The listing builds one solid part. Answer for the finished solid, in the listing's coordinates (mm). A direction names the side the tool comes from. Coordinates: 2 decimals unless noted, no trailing zeros. Loops run counter-clockwise (first coordinate to the right, second up) from the corner with the lowest first, then second, coordinate; pieces in that order, holes last. Notation, with made-up numbers: (-38.5, 1.25) -> (-29.5, 1.25) arc R21 cw to (-29.5, 13.25) -> close; hole circle Ø10 at (67, 5). An arc over 180 degrees is marked (long way). Answer in a Markdown table with one row per item.
```python
from build123d import *

# Parameters (mm, degrees)
PAD016_DEPTH         = 27.5
POCKET034_DEPTH      = 185.6284208373
SKETCH105_W          = 70
SKETCH105_H          = 70
POCKET036_DEPTH      = 2.501
SKETCH114_W          = 70
SKETCH114_H          = 16
POCKET051_DEPTH      = 30.601
POCKET051_DEPTH_BACK = 30.601
PAD020_DEPTH         = 5
SKETCH134_R          = 2.3
SKETCH135_R          = 4
POCKET052_DEPTH      = 9
POCKET053_DEPTH      = 0.001
POCKET053_DEPTH_BACK = 22.501
SKETCH138_R          = 6.5
POCKET054_DEPTH      = 12.8357525158
POCKET056_DEPTH      = 2.5010001


with BuildPart() as part:
    # Sketch096 → Pad016 (new body)
    with BuildSketch(Plane.XY.offset(2.5)):
        with BuildLine():
            Line((-22.6, 30.6), (22.6, 30.6))
            ThreePointArc((30.6, 22.6), (28.2568542495, 28.2568542495), (22.6, 30.6))
            Line((30.6, 22.6), (30.6, -22.6))
            ThreePointArc((22.6, -30.6), (28.2568542495, -28.2568542495), (30.6, -22.6))
            Line((22.6, -30.6), (-22.6, -30.6))
            ThreePointArc((-30.6, -22.6), (-28.2568542495, -28.2568542495), (-22.6, -30.6))
            Line((-30.6, -22.6), (-30.6, 22.6))
            ThreePointArc((-22.6, 30.6), (-28.2568542495, 28.2568542495), (-30.6, 22.6))
        make_face()
    extrude(amount=-PAD016_DEPTH)

    # Sketch103 → Pocket034 (cut, through all)
    with BuildSketch(Plane.XY.offset(-1.5)):
        with BuildLine():
            Line((14.1, 7.65), (20.4, 7.65))
            ThreePointArc((21.9, 6.15), (21.4606601718, 7.2106601718), (20.4, 7.65))
            Line((21.9, 6.15), (21.9, -6.15))
            ThreePointArc((20.4, -7.65), (21.4606601718, -7.2106601718), (21.9, -6.15))
            Line((20.4, -7.65), (14.1, -7.65))
            ThreePointArc((12.6, -6.15), (13.0393398282, -7.2106601718), (14.1, -7.65))
            Line((12.6, -6.15), (12.6, 6.15))
            ThreePointArc((14.1, 7.65), (13.0393398282, 7.2106601718), (12.6, 6.15))
        make_face()
    pocket034 = extrude(amount=POCKET034_DEPTH, mode=Mode.SUBTRACT)

    # Mirrored008: Pocket034 across YZ
    add(pocket034.mirror(Plane.YZ), mode=Mode.SUBTRACT)

    # Sketch105 → Pocket036 (cut, through all)
    with BuildSketch(Plane.XY):
        Rectangle(SKETCH105_W, SKETCH105_H)
        with BuildLine():
            Line((-22.8, 25.9), (22.8, 25.9))
            ThreePointArc((26.3, 22.4), (25.2748737342, 24.8748737342), (22.8, 25.9))
            Line((26.3, 22.4), (26.3, -22.4))
            ThreePointArc((22.8, -25.9), (25.2748737342, -24.8748737342), (26.3, -22.4))
            Line((22.8, -25.9), (-22.8, -25.9))
            ThreePointArc((-26.3, -22.4), (-25.2748737342, -24.8748737342), (-22.8, -25.9))
            Line((-26.3, -22.4), (-26.3, 22.4))
            ThreePointArc((-22.8, 25.9), (-25.2748737342, 24.8748737342), (-26.3, 22.4))
        make_face(mode=Mode.SUBTRACT)
    extrude(amount=POCKET036_DEPTH, mode=Mode.SUBTRACT)

    # Sketch107 → Groove012 (revolve, cut)
    with BuildSketch(Plane.XZ):
        Polygon((19, -1.5), (21.8, -1.5), (21.2, -3.1484864517), (21.2, -13.5), (19, -13.5), align=None)
    groove012 = revolve(axis=Axis((19, 0, -1.5), (0, 0, 1)), mode=Mode.SUBTRACT)

    # Mirrored009: Groove012 across YZ
    add(groove012.mirror(Plane.YZ), mode=Mode.SUBTRACT)

    # Sketch114 → Pocket051 (cut, two sides)
    with BuildSketch(Plane.XZ) as pocket051_sk:
        with Locations((0, -18)):
            Rectangle(SKETCH114_W, SKETCH114_H)
    extrude(amount=-POCKET051_DEPTH, mode=Mode.SUBTRACT)
    extrude(pocket051_sk.sketch, amount=POCKET051_DEPTH_BACK, mode=Mode.SUBTRACT)

    # AdditivePipe004: sweep along a path in Sketch130
    with BuildLine(Plane.XY) as additivepipe004_path:
        Line((27, 16), (27, -5))
        ThreePointArc((27, -5), (25.1488749734, -9.9623583103), (20.5, -12.5))
        ThreePointArc((20.5, -12.5), (15.8511250266, -15.0376416897), (14, -20))
        Line((14, -20), (14, -30.6))
    # Sketch131 → AdditivePipe004 (sweep)
    with BuildSketch(Plane.XZ):
        with BuildLine():
            ThreePointArc((29.037037037, -18.5506966813), (27, -17.5), (24.962962963, -18.5506966813))
            ThreePointArc((24.6, -18.4347524158), (24.7391419381, -18.6252682846), (24.962962963, -18.5506966813))
            Line((24.6, -10), (24.6, -18.4347524158))
            Line((29.4, -10), (24.6, -10))
            Line((29.4, -18.4347524157), (29.4, -10))
            ThreePointArc((29.037037037, -18.5506966812), (29.2608580619, -18.6252682846), (29.4, -18.4347524157))
        make_face()
    sweep(path=additivepipe004_path.line)

    # Sketch110 → Pad020 (join)
    with BuildSketch(Plane.XZ.offset(30.6)):
        with BuildLine():
            ThreePointArc((-8.85, -18.1), (-9.4228261259, -18.2136846573), (-9.9088235294, -18.5375063607))
            ThreePointArc((-10.25, -18.3958405421), (-10.1266964989, -18.5805501712), (-9.9088235294, -18.5375063607))
            Line((-10.25, -10), (-10.25, -18.3958405421))
            Line((-2.25, -10), (-10.25, -10))
            Line((-2.25, -18.3958405421), (-2.25, -10))
            ThreePointArc((-2.5911764706, -18.5375063607), (-2.3733035011, -18.5805501712), (-2.25, -18.3958405421))
            ThreePointArc((-2.5911764706, -18.5375063607), (-3.0771738741, -18.2136846573), (-3.65, -18.1))
            Line((-8.85, -18.1), (-3.65, -18.1))
        make_face()
    extrude(amount=-PAD020_DEPTH)

    # Sketch134 → AdditiveLoft section 0
    with BuildSketch(Plane.XY.offset(-17.5)):
        with Locations((-6, -6.5)):
            Circle(SKETCH134_R)
    # Sketch135 → AdditiveLoft section 1
    with BuildSketch(Plane.XY.offset(-10)):
        with Locations((-6, -6.5)):
            Circle(SKETCH135_R)
    loft()

    # AdditivePipe005: sweep along a path in Sketch136
    with BuildLine(Plane.XY) as additivepipe005_path:
        Line((-22.5, 29.5), (22.5, 29.5))
        ThreePointArc((22.5, 29.5), (27.4497474683, 27.4497474683), (29.5, 22.5))
        Line((29.5, 22.5), (29.5, -22.5))
        ThreePointArc((29.5, -22.5), (27.4497474683, -27.4497474683), (22.5, -29.5))
        Line((22.5, -29.5), (-22.5, -29.5))
        ThreePointArc((-22.5, -29.5), (-27.4497474683, -27.4497474683), (-29.5, -22.5))
        Line((-29.5, -22.5), (-29.5, 22.5))
        ThreePointArc((-29.5, 22.5), (-27.4497474683, 27.4497474683), (-22.5, 29.5))
    # Sketch137 → AdditivePipe005 (sweep)
    with BuildSketch(Plane.YZ):
        Polygon((30.3970562748, -10), (28.6029437252, -10), (29.1, -11.2), (29.9, -11.2), align=None)
    sweep(path=additivepipe005_path.line)

    # Sketch104 → Pocket052 (cut, symmetric)
    with BuildSketch(Plane.XY.offset(-11)):
        Polygon((-26.5, 27), (17.5, 27), (17.5, 23), (15.5, 23), (15.5, 7), (-25.5, 7), (-25.5, 23), (-26.5, 23), align=None)
    extrude(amount=POCKET052_DEPTH, both=True, mode=Mode.SUBTRACT)

    # Sketch099 → Groove018 (revolve, cut)
    with BuildSketch(Plane.XZ.offset(8)):
        Polygon((-26, 3), (-26, -24), (-24.2, -24), (-24.2, -8), (-23, -6.8), (-23, 3), align=None)
    revolve(axis=Axis((-26, -8, 3), (0, 0, 1)), mode=Mode.SUBTRACT)

    # Sketch100 → Groove019 (revolve, cut)
    with BuildSketch(Plane.XZ.offset(25)):
        Polygon((25, 3), (25, -24), (26.8, -24), (26.8, -8), (28, -6.8), (28, 3), align=None)
    revolve(axis=Axis((25, -25, 3), (0, 0, 1)), mode=Mode.SUBTRACT)

    # Sketch101 → Groove020 (revolve, cut)
    with BuildSketch(Plane.XZ.offset(-25)):
        Polygon((25, 3), (25, -24), (26.8, -24), (26.8, -8), (28, -6.8), (28, 3), align=None)
    revolve(axis=Axis((25, 25, 3), (0, 0, 1)), mode=Mode.SUBTRACT)

    # Sketch113 → Pocket053 (cut, two sides)
    with BuildSketch(Plane.XY.offset(-20)) as pocket053_sk:
        with BuildLine():
            ThreePointArc((22.8349364905, 22.25), (23.8543560763, 21.6928108612), (25, 21.5))
            ThreePointArc((27, 19.5), (26.4142135624, 20.9142135624), (25, 21.5))
            Line((27, 9.5), (27, 19.5))
            ThreePointArc((23.5, 6), (25.9748737342, 7.0251262658), (27, 9.5))
            Line((9.5, 6), (23.5, 6))
            ThreePointArc((6, 9.5), (7.0251262658, 7.0251262658), (9.5, 6))
            Line((6, 19.5), (6, 9.5))
            ThreePointArc((9.5, 23), (7.0251262658, 21.9748737342), (6, 19.5))
            Line((20.6698729811, 23), (9.5, 23))
            ThreePointArc((22.8349364905, 22.25), (21.8155169048, 22.8071891388), (20.6698729811, 23))
        make_face()
    extrude(amount=-POCKET053_DEPTH, mode=Mode.SUBTRACT)
    extrude(pocket053_sk.sketch, amount=POCKET053_DEPTH_BACK, mode=Mode.SUBTRACT)

    # Sketch138 → Pocket054 (cut, through all)
    with BuildSketch(Plane.XY.offset(-5.8)):
        with Locations((19, 0)):
            Circle(SKETCH138_R)
        with Locations((-19, 0)):
            Circle(SKETCH138_R)
    extrude(amount=-POCKET054_DEPTH, mode=Mode.SUBTRACT)

    # Sketch144 → Pocket056 (cut, through all)
    with BuildSketch(Plane.XY):
        with BuildLine():
            Line((-8.5, 23), (8.5, 23))
            ThreePointArc((11.5, 20), (10.6213203436, 22.1213203436), (8.5, 23))
            Line((11.5, 20), (11.5, -20))
            ThreePointArc((8.5, -23), (10.6213203436, -22.1213203436), (11.5, -20))
            Line((8.5, -23), (-8.5, -23))
            ThreePointArc((-11.5, -20), (-10.6213203436, -22.1213203436), (-8.5, -23))
            Line((-11.5, -20), (-11.5, 20))
            ThreePointArc((-8.5, 23), (-10.6213203436, 22.1213203436), (-11.5, 20))
        make_face()
    extrude(amount=POCKET056_DEPTH, mode=Mode.SUBTRACT)


solid = part.part
```
Item 1: Find the intervals of material crossed by probe 1 along Y at (x, z) = (19, -5.2); probe 2 along Y at (x, z) = (-19, -7.7); probe 3 along Y at (x, z) = (19, 0.75), in increasing order.
Findings below:
| item | result |
|---|---|
| probe 1 | y = -30.6 to -2.2, 2.2 to 6, 23 to 30.6 |
| probe 2 | y = -30.6 to -6.5, 6.5 to 7, 27 to 30.6 |
| probe 3 | y = -25.9 to -7.65, 23 to 25.9 |
Item 2: A cutting plane is placed at B-B, the plane y = 0. Count the separate pieces of the cut face and the enclosed holes in it, plus the area to 3 significant figures.
Findings below:
| item | result |
|---|---|
| separate pieces | 3 |
| enclosed holes | 0 |
| area | 496 mm2 |
Item 3: A cutting plane is placed at A-A, the plane x = -6. Determine the outline of the cut face in (y, z).
Findings below:
| item | result |
|---|---|
| outline | (-30.6, -18.1) -> (-25.6, -18.1) -> (-25.6, -10) -> (-10.5, -10) -> (-8.8, -17.5) -> (-4.2, -17.5) -> (-2.5, -10) -> (7, -10) -> (7, -2) -> (27, -2) -> (27, -10) -> (28.6, -10) -> (29.1, -11.2) -> (29.9, -11.2) -> (30.4, -10) -> (30.6, -10) -> (30.6, 0) -> (25.9, 0) -> (25.9, 2.5) -> (23, 2.5) -> (23, 0) -> (-23, 0) -> (-23, 2.5) -> (-25.9, 2.5) -> (-25.9, 0) -> (-30.6, 0) -> close |
Item 4: A tool of negligible diameter and unlimited length cuts with its end or side. For faces 5 (the face through (26.96, -26.87, -10.34)), 6 (the face through (16, 6, -5)), 7 (the face through (-1, 25.9, 1)), 8 (the face through (-17, -7.65, 0)), 9 (the face through (-6, -28, -18.1)), from which of +Z, -Z, +X, -X, +Y, -Y can it reach the whole face along a straight path? Write none if from no direction.
Findings below:
| item | result |
|---|---|
| face 5 | -Z |
| face 6 | +Z, -Z |
| face 7 | +Z, +X, -X, +Y |
| face 8 | +Z |
| face 9 | -Z, +Y, -Y |
Item 5: Determine the mould class of faces 1 (the face through (-28.194, 28.319, -4.93)), 2 (the face through (-28.319, -28.194, -4.93)), 3 (the face through (7.524, 22.389, -0.782)), 4 (the face through (14, -25.4, -17.5)) for opening direction Y: +Y half, -Y half, draft (parallel to the pull), parting line (faces both ways), or undercut.
Findings below:
| item | result |
|---|---|
| face 1 | +Y half |
| face 2 | -Y half |
| face 3 | undercut |
| face 4 | draft |
Item 6: Flat-ended cylindrical pins translate along their axes: pin 1 Ø4 at (x, y) = (-20, 2.5) entering from -Z; pin 2 Ø0.9 at (x, y) = (22.5, 5) entering from -Z; pin 3 Ø4 at (x, z) = (-6, -13.5) entering from +Y. Find the tip coordinate at first contact, or state that the pin passes through.
Findings below:
| item | result |
|---|---|
| pin 1 | stops at z = -5.8 |
| pin 2 | stops at z = -10 |
| pin 3 | stops at y = -2.84 |
Item 7: A cutting plane is placed at C-C, the plane x = 1. Determine the outline of the cut face in (y, z).
Findings below:
| item | result |
|---|---|
| outline | (-30.6, -10) -> (-30.4, -10) -> (-29.9, -11.2) -> (-29.1, -11.2) -> (-28.6, -10) -> (7, -10) -> (7, -2) -> (27, -2) -> (27, -10) -> (28.6, -10) -> (29.1, -11.2) -> (29.9, -11.2) -> (30.4, -10) -> (30.6, -10) -> (30.6, 0) -> (25.9, 0) -> (25.9, 2.5) -> (23, 2.5) -> (23, 0) -> (-23, 0) -> (-23, 2.5) -> (-25.9, 2.5) -> (-25.9, 0) -> (-30.6, 0) -> close |
